```python
from build123d import *

# Parameters (mm, degrees)
SKIZZE1_W                       = 151
SKIZZE1_H                       = 55
AUFSATZ_LINEAR_AUSTRAGEN1_DEPTH = 3
SKIZZE2_R                       = 11
SCHNITT_LINEAR_AUSTRAGEN1_DEPTH = 17
SKIZZE3_R                       = 1.5
SCHNITT_LINEAR_AUSTRAGEN2_DEPTH = 10
SKIZZE4_R                       = 4
SCHNITT_LINEAR_AUSTRAGEN3_DEPTH = 10
SKIZZE5_R                       = 2
SCHNITT_LINEAR_AUSTRAGEN4_DEPTH = 10


with BuildPart() as part:
    # Skizze1 → Aufsatz-Linear austragen1 (new body)
    with BuildSketch(Plane.XY):
        with Locations((75.5, 27.5)):
            Rectangle(SKIZZE1_W, SKIZZE1_H)
    extrude(amount=AUFSATZ_LINEAR_AUSTRAGEN1_DEPTH)

    # Skizze2 → Schnitt-Linear austragen1 (cut)
    with BuildSketch(Plane.XY.offset(3)):
        with Locations((75.5, 34)):
            Circle(SKIZZE2_R)
    extrude(amount=-SCHNITT_LINEAR_AUSTRAGEN1_DEPTH, mode=Mode.SUBTRACT)

    # Skizze3 → Schnitt-Linear austragen2 (cut)
    with BuildSketch(Plane.XY.offset(3)):
        with Locations((91, 49.5)):
            Circle(SKIZZE3_R)
        with Locations((91, 18.5)):
            Circle(SKIZZE3_R)
        with Locations((60, 18.5)):
            Circle(SKIZZE3_R)
        with Locations((60, 49.5)):
            Circle(SKIZZE3_R)
    extrude(amount=-SCHNITT_LINEAR_AUSTRAGEN2_DEPTH, mode=Mode.SUBTRACT)

    # Skizze4 → Schnitt-Linear austragen3 (cut)
    with BuildSketch(Plane.XY.offset(3)):
        with Locations((141, 30)):
            Circle(SKIZZE4_R)
        with Locations((10, 30)):
            Circle(SKIZZE4_R)
    extrude(amount=-SCHNITT_LINEAR_AUSTRAGEN3_DEPTH, mode=Mode.SUBTRACT)

    # Skizze5 → Schnitt-Linear austragen4 (cut)
    with BuildSketch(Plane.XY.offset(3)):
        with Locations((10, 10)):
            Circle(SKIZZE5_R)
        with Locations((55, 10)):
            Circle(SKIZZE5_R)
        with Locations((96, 10)):
            Circle(SKIZZE5_R)
        with Locations((141, 10)):
            Circle(SKIZZE5_R)
    extrude(amount=-SCHNITT_LINEAR_AUSTRAGEN4_DEPTH, mode=Mode.SUBTRACT)


solid = part.part
```
CAD build for the part. Positions are in the model's coordinates, mm. Round coordinates to 2 decimals unless told otherwise and drop trailing zeros. Order: outer loops, then holes, each group sorted by start corner. A loop starts at its lowest first (then second) coordinate and runs counter-clockwise, first axis right, second up. Notation, with made-up numbers: (-38, 16) -> (-32, 16) arc R23 cw to (-32, 40) -> close; hole circle Ø4 at (-32, -5.5). An arc over 180 degrees is marked (long way). One line per question, with ' | ' between items.
Q1. Slice it at B-B (y = 10). Write the cut outline in (x, z), then the cut area to 3 significant figures.
Completed:
outline: (0, 0) -> (8, 0) -> (8, 3) -> (0, 3) -> close; (12, 0) -> (53, 0) -> (53, 3) -> (12, 3) -> close; (57, 0) -> (94, 0) -> (94, 3) -> (57, 3) -> close; (98, 0) -> (139, 0) -> (139, 3) -> (98, 3) -> close; (143, 0) -> (151, 0) -> (151, 3) -> (143, 3) -> close | area: 405 mm^2
Q2. Slice it at C-C (z = 0.55). Give the number of separate pieces and of enclosed holes in the cut face, then the cut area to 3 significant figures.
Completed:
separate pieces: 1 | enclosed holes: 11 | area: 7,750 mm^2
Q3. Slice it at A-A (x = 55). Write the cut outline in (y, z), then the cut area to 3 significant figures.
Completed:
outline: (0, 0) -> (8, 0) -> (8, 3) -> (0, 3) -> close; (12, 0) -> (55, 0) -> (55, 3) -> (12, 3) -> close | area: 153 mm^2
Q4. Slice it at D-D (y = 49.5). Write the cut outline in (x, z), then the cut area to 3 significant figures.
Completed:
outline: (0, 0) -> (58.5, 0) -> (58.5, 3) -> (0, 3) -> close; (61.5, 0) -> (89.5, 0) -> (89.5, 3) -> (61.5, 3) -> close; (92.5, 0) -> (151, 0) -> (151, 3) -> (92.5, 3) -> close | area: 435 mm^2
Q5. Probe probe 1 along Y at (x, z) = (91, 1.6); probe 2 along Y at (x, z) = (96, 0.75); probe 3 along Y at (x, z) = (139.5, 1.75). List the from-to ranges inside material, lowest first.
Completed:
probe 1: y = 0 to 17, 20 to 48, 51 to 55 | probe 2: y = 0 to 8, 12 to 55 | probe 3: y = 0 to 8.68, 11.32 to 26.29, 33.71 to 55
Q6. Two-plate mould, pull along Y, no slides. Class faces 1 (the cylindrical face through (64.51, 34.48, 1.52)), 2 (the flat face through (74, 55, 1)), 3 (the cylindrical face through (60.69, 48.17, 1.52)), 4 (the flat face through (0, 27, 1)): released by +Y, released by -Y, zero draft, split by the parting line, or undercut.
Completed:
face 1: undercut | face 2: released by +Y | face 3: undercut | face 4: zero draft
